Input: part model. Units: mm. Frame: model coordinates. A direction names the side the tool comes from. Coordinates: 2 decimals unless noted, no trailing zeros. Write each loop counter-clockwise with the first axis right and the second up, starting at its lowest first coordinate (ties: lowest second). Pieces come first, ordered by that corner, then holes. Notation, with made-up numbers: (-6.5, -10) - (45.5, -10) arc R29 cw to (45.5, 15) - close; hole circle Ø5 at (-29, 49.25). An arc over 180 degrees is marked (long way). Put each result on its own line as item: value. Start each with the question number.
1. Pull-direction query (X, two-part tool) for faces 4 (the flat face through (59, 3, -5.676)), 5 (the flat face through (49.213, 3, -59)), 6 (the flat face through (28.55, 3, -50)), 7 (the flat face through (45.282, 3, -17)); classes: released by +X, released by -X, zero draft, split by the parting line, or undercut.
2. Line query: line 1 (Z direction, x = 55.5, y = 3.25); line 2 (Z direction, x = 11, y = 0.5) (1 decimal); line 3 (Z direction, x = 59, y = 3.5). Output: solid intervals per line, ascending.
3. Access query for faces 1 (the flat face through (54, 3, -54.888)), 2 (the flat face through (51, 3, -56.476)), 3 (the flat face through (26, 3, -39.688)). Directions: +Z, -Z, +X, -X, +Y, -Y. A direction counts if a zero-diameter tool reaches every point of the face in a straight line with its end or side. Return the directions, or none.
4. Cut plane A-A, the plane x = 27. Count the separate pieces of the cut face and the enclosed holes in it, and give its area (3 significant figures).
5. Cut plane B-B, the plane x = 47. Return loops of the section in (y, z).
6. Pin query (flat end, axial travel): pin 1 (3 mm diameter, centred on x = 35, y = 3, fed in from +Z). Return the tip coordinate at first contact, or that it passes through.
7. Cut plane D-D, the plane z = -9. Return loops of the section in (x, y), and give its area (4 significant figures).
from build123d import *

# Parameters (mm, degrees)
BOSS_EXTRUDE1_DEPTH = 6.35
SKETCH2_W           = 6.35
SKETCH2_H           = 1.5875
CUT_EXTRUDE1_DEPTH  = 6.35
BOSS_EXTRUDE2_START = -6.35
SKETCH4_W           = 24.326613467
SKETCH4_H           = 69.85
BOSS_EXTRUDE2_DEPTH = 6.35
SKETCH5_W           = 25.4
SKETCH5_H           = 3.175
CUT_EXTRUDE3_DEPTH  = 6.35
SKETCH7_W           = 19.923596682
SKETCH7_H           = 95.25
CUT_EXTRUDE4_DEPTH  = 6.35
SKETCH8_W           = 15.043251586
SKETCH8_H           = 69.85
CUT_EXTRUDE5_DEPTH  = 6.35
SKETCH9_W           = 3.175
SKETCH9_H           = 95.25
BOSS_EXTRUDE3_DEPTH = 6.35
SKETCH10_W          = 17.539756693
SKETCH10_H          = 95.25
CUT_EXTRUDE7_DEPTH  = 6.35
SKETCH3_W           = 4.7625
SKETCH3_H           = 14.2875
SKETCH3_W_2         = 9.525
SKETCH3_H_2         = 3.175
CUT_EXTRUDE8_DEPTH  = 6.35
SKETCH11_W          = 14.2875
SKETCH11_H          = 4.7625
SKETCH11_W_2        = 3.175
SKETCH11_H_2        = 7.9375
CUT_EXTRUDE9_DEPTH  = 6.35
SKETCH13_W          = 15.043251586
SKETCH13_H          = 51.369192813
BOSS_EXTRUDE4_DEPTH = 6.35
SKETCH14_W          = 14.2875
SKETCH14_H          = 4.7625
SKETCH14_W_2        = 3.175
SKETCH14_H_2        = 7.9375
CUT_EXTRUDE10_DEPTH = 6.35


with BuildPart() as part:
    # Sketch1 → Boss-Extrude1 (new body)
    with BuildSketch(Plane(origin=(0, 0, 0), x_dir=(1, 0, 0), z_dir=(0, 1, 0))):
        Polygon((38.1, 65.0875), (84.214756693, 65.0875), (84.214756693, -30.1625), (38.1, -30.1625), (38.1, -19.05), (19.05, -19.05), (19.05, -25.4), (6.35, -25.4), (6.35, -19.05), (0, -19.05), (0, 0), (0, 34.925), (0, 53.975), (6.35, 53.975), (6.35, 60.325), (19.05, 60.325), (19.05, 53.975), (38.1, 53.975), align=None)
        Polygon((38.1, 34.925), (44.45, 38.591174209), (44.45, 52.3875), (74.689756693, 52.3875), (77.864756693, 50.8), (77.864756693, -15.875), (74.689756693, -17.4625), (44.45, -17.4625), (44.45, -3.666174209), (38.1, 0), align=None, mode=Mode.SUBTRACT)
    extrude(amount=BOSS_EXTRUDE1_DEPTH)

    # Sketch2 → Cut-Extrude1 (cut)
    with BuildSketch(Plane(origin=(0, 6.35, 0), x_dir=(1, 0, 0), z_dir=(0, 1, 0))):
        with Locations((9.525, 35.71875)):
            Rectangle(SKETCH2_W, SKETCH2_H)
        with Locations((9.525, -0.79375)):
            Rectangle(SKETCH2_W, SKETCH2_H)
        with Locations((28.575, 35.71875)):
            Rectangle(SKETCH2_W, SKETCH2_H)
        with Locations((28.575, -0.79375)):
            Rectangle(SKETCH2_W, SKETCH2_H)
    extrude(amount=-CUT_EXTRUDE1_DEPTH, mode=Mode.SUBTRACT)

    # Sketch4 → Boss-Extrude2 (add)
    with BuildSketch(Plane(origin=(0, 6.35, 0), x_dir=(1, 0, 0), z_dir=(0, 1, 0)).offset(BOSS_EXTRUDE2_START)):
        with Locations((49.82644996, 17.4625)):
            Rectangle(SKETCH4_W, SKETCH4_H)
    extrude(amount=BOSS_EXTRUDE2_DEPTH)

    # Sketch5 → Cut-Extrude3 (cut)
    with BuildSketch(Plane(origin=(0, 6.35, 0), x_dir=(1, 0, 0), z_dir=(0, 1, 0))):
        with Locations((61.989756693, 17.4625)):
            Rectangle(SKETCH5_W, SKETCH5_H)
        with Locations((36.589756693, 17.4625)):
            Rectangle(SKETCH5_W, SKETCH5_H)
    extrude(amount=-CUT_EXTRUDE3_DEPTH, mode=Mode.SUBTRACT)

    # Sketch7 → Cut-Extrude4 (cut)
    with BuildSketch(Plane(origin=(0, 6.35, 0), x_dir=(1, 0, 0), z_dir=(0, 1, 0))):
        with Locations((91.001555034, 17.4625)):
            Rectangle(SKETCH7_W, SKETCH7_H)
    extrude(amount=-CUT_EXTRUDE4_DEPTH, mode=Mode.SUBTRACT)

    # Sketch8 → Cut-Extrude5 (cut)
    with BuildSketch(Plane.XZ):
        with Locations((52.803374207, -17.4625)):
            Rectangle(SKETCH8_W, SKETCH8_H)
    extrude(amount=-CUT_EXTRUDE5_DEPTH, mode=Mode.SUBTRACT)

    # Sketch9 → Boss-Extrude3 (add)
    with BuildSketch(Plane.XZ):
        with Locations((61.9125, -17.4625)):
            Rectangle(SKETCH9_W, SKETCH9_H)
    extrude(amount=-BOSS_EXTRUDE3_DEPTH)

    # Sketch10 → Cut-Extrude7 (cut)
    with BuildSketch(Plane.XZ):
        with Locations((72.269878347, -17.4625)):
            Rectangle(SKETCH10_W, SKETCH10_H)
    extrude(amount=-CUT_EXTRUDE7_DEPTH, mode=Mode.SUBTRACT)

    # Sketch3 → Cut-Extrude8 (cut)
    with BuildSketch(Plane(origin=(0, 6.35, 0), x_dir=(1, 0, 0), z_dir=(0, 1, 0))):
        with Locations((26.168267374, 46.83125)):
            Rectangle(SKETCH3_W, SKETCH3_H)
        with Locations((26.168267374, 44.45)):
            Rectangle(SKETCH3_W_2, SKETCH3_H_2)
        with Locations((26.168267374, -9.525)):
            Rectangle(SKETCH3_W_2, SKETCH3_H_2)
        with Locations((26.168267374, -11.90625)):
            Rectangle(SKETCH3_W, SKETCH3_H)
    extrude(amount=-CUT_EXTRUDE8_DEPTH, mode=Mode.SUBTRACT)

    # Sketch11 → Cut-Extrude9 (cut)
    with BuildSketch(Plane.XZ):
        with Locations((56.35625, 23.932056084)):
            Rectangle(SKETCH11_W, SKETCH11_H)
        with Locations((53.975, 23.932056084)):
            Rectangle(SKETCH11_W_2, SKETCH11_H_2)
        with Locations((53.975, -58.857056084)):
            Rectangle(SKETCH11_W_2, SKETCH11_H_2)
        with Locations((56.35625, -58.857056084)):
            Rectangle(SKETCH11_W, SKETCH11_H)
    extrude(amount=-CUT_EXTRUDE9_DEPTH, mode=Mode.SUBTRACT)

    # Sketch13 → Boss-Extrude4 (add)
    with BuildSketch(Plane.XZ):
        with Locations((52.803374207, -26.702903594)):
            Rectangle(SKETCH13_W, SKETCH13_H)
    extrude(amount=-BOSS_EXTRUDE4_DEPTH)

    # Sketch14 → Cut-Extrude10 (cut)
    with BuildSketch(Plane.XZ):
        with Locations((56.35625, -8.057056084)):
            Rectangle(SKETCH14_W, SKETCH14_H)
        with Locations((53.975, -8.057056084)):
            Rectangle(SKETCH14_W_2, SKETCH14_H_2)
    extrude(amount=-CUT_EXTRUDE10_DEPTH, mode=Mode.SUBTRACT)


solid = part.part
Report:
1. face 4: zero draft
1. face 5: released by +X
1. face 6: undercut
1. face 7: undercut
2. line 1: z = -65.09 to -62.83, -54.89 to -12.03, -4.09 to -1.02, 17.46 to 19.96, 27.9 to 30.16
2. line 2: z = -60.3 to -36.5, -34.9 to 0, 1.6 to 25.4
2. line 3: z = -65.09 to -61.24, -56.48 to -10.44, -5.68 to -1.02, 17.46 to 21.55, 26.31 to 30.16
3. face 1: +Y, -Y
3. face 2: +X, +Y, -Y
3. face 3: -Z, +Y, -Y
4. separate pieces: 4
4. enclosed holes: 0
4. area: 242 mm^2
5. outline: (0, -65.09) - (6.35, -65.09) - (6.35, -1.02) - (0, -1.02) - close; (0, 17.46) - (6.35, 17.46) - (6.35, 30.16) - (0, 30.16) - close
6. pin 1: stops at z = 19.05
7. outline: (0, 0) - (49.21, 0) - (49.21, 6.35) - (0, 6.35) - close
7. area: 312.5 mm^2
